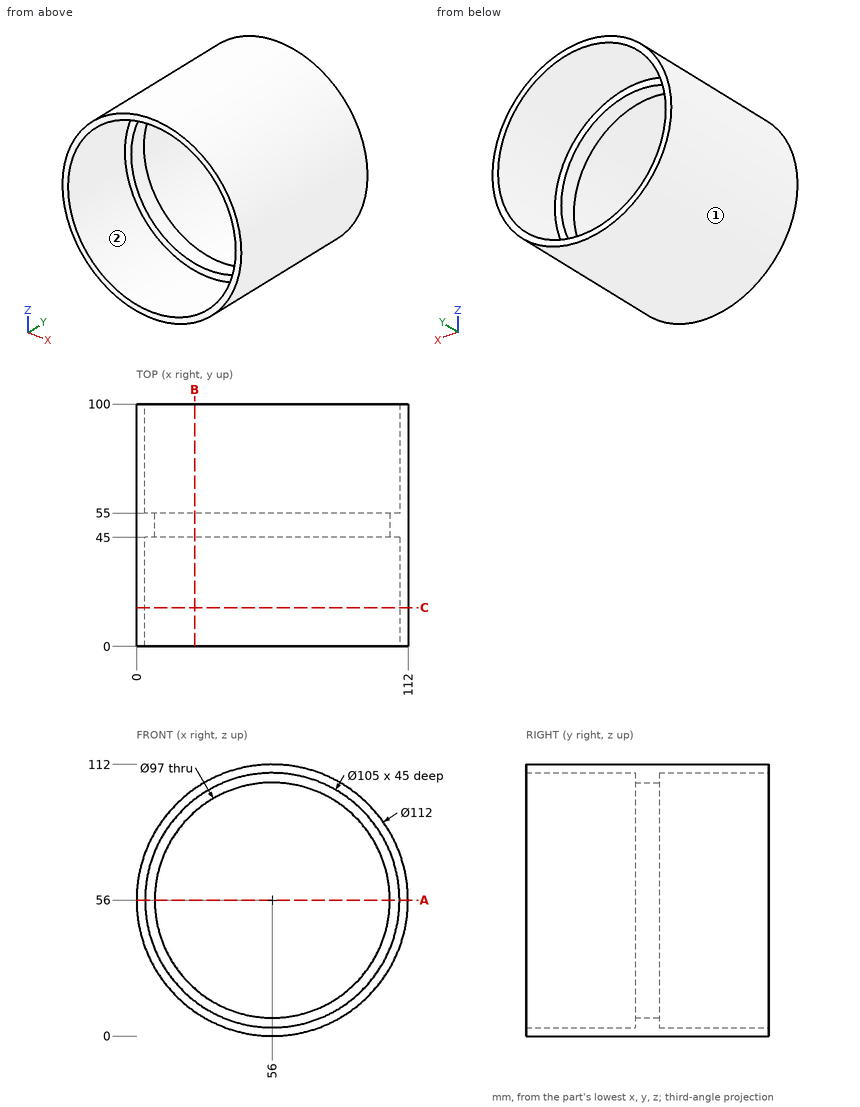
Could you check a few things on this drawing? It's one solid part, dimensions in mm from its lowest x, y, z. Give positions to 0.01 mm unless a question says otherwise; leave off trailing zeros. Order: outer loops, then holes, each group sorted by start corner. A loop starts at its lowest first (then second) coordinate and runs counter-clockwise, first axis right, second up. Notation, with made-up numbers: (18.5, 29) - (74.5, 29) arc R8 ccw to (74.5, 43) - close; hole circle Ø1 at (83, -25.75). An arc over 180 degrees is marked (long way). Answer as a JSON object with one key per item and string values. Group by question number.
Item 1: If we mould it in two halves opening along Z, with no side actions, what happens to the marked faces 1 and 2? For each: pulls with the +Z half, pulls with the -Z half, needs draft (parallel to the pull), parting line crosses it, or undercut.
Item 2: For P1, Ø10, axis at x = 60.5, y = 71.5, coming from the +Z side; P2, Ø1, axis at x = 24.5, y = 70, coming from the -Z side; P3, Ø12, axis at y = 21.5, z = 48.5, coming from the +X side; P4, Ø12, axis at x = 14.5, z = 52.5, coming from the -Y side, each with a flat end and sliding along its axis, tell me the tip position at first contact or that it passes through.
Item 3: If we section it at A-A on z = 56: Please give me the cut outline in (x, y), and give its area (3 significant figures).
Item 4: If we section it at C-C on y = 16: Please give me the cut outline in (x, z).
Item 5: If we section it at B-B on x = 24: Please give me the cut outline in (y, z).
Item 6: Please list where these lines run through material, in increasing order: probe 1 along Z at (x, y) = (56, 51.75); probe 2 along Z at (x, y) = (56, 27); probe 3 along X at (y, z) = (79, 99).
Result set:
{
 "1": {"face 1": "parting line crosses it", "face 2": "undercut"},
 "2": {"P1": "z = 112", "P2": "z = 9.36", "P3": "x = 111.98", "P4": "through"},
 "3": {"outline": "(0, 0) - (3.5, 0) - (3.5, 45) - (7.5, 45) - (7.5, 55) - (3.5, 55) - (3.5, 100) - (0, 100) - close; (104.5, 45) - (108.5, 45) - (108.5, 0) - (112, 0) - (112, 100) - (108.5, 100) - (108.5, 55) - (104.5, 55) - close", "area": "780 mm²"},
 "4": {"outline": "circle Ø112 at (56, 56); hole circle Ø105 at (56, 56)"},
 "5": {"outline": "(0, 10.04) - (100, 10.04) - (100, 14.38) - (55, 14.38) - (55, 19.55) - (45, 19.55) - (45, 14.38) - (0, 14.38) - close; (0, 97.62) - (45, 97.62) - (45, 92.45) - (55, 92.45) - (55, 97.62) - (100, 97.62) - (100, 101.96) - (0, 101.96) - close"},
 "6": {"probe 1": "0 to 7.5, 104.5 to 112", "probe 2": "0 to 3.5, 108.5 to 112", "probe 3": "20.13 to 25.88, 86.12 to 91.87"}
}
